The drawing under review shows one solid part. Ordinate dimensions are in mm from its lowest x, y, z. Coordinates: 2 decimals unless noted, no trailing zeros. Order: outer loops, then holes, each group sorted by start corner. A loop starts at its lowest first (then second) coordinate and runs counter-clockwise, first axis right, second up. Notation, with made-up numbers: (4, 69) -> (27, 69) arc R28 cw to (27, 97) -> close; hole circle Ø8 at (-30.5, -22). An arc over 180 degrees is marked (long way). Use a Markdown table: item, result. Add a question column.
Q1. Wall thickness on probe 1 along X at (y, z) = (35.5, 3.75); probe 2 along Y at (x, z) = (56.5, 2.95); probe 3 along Y at (x, z) = (46, 3.3): over which ranges is each line inside the solid? List them lowest first.
Q2. Insertion check: pin 1 (2.5 mm diameter, centred on x = 57, z = 2, fed in from +Y); pin 2 (1 mm diameter, centred on x = 13, z = 3, fed in from +Y); pin 3 (5 mm diameter, centred on x = 29, y = 99, fed in from -Z). Each pin has a flat end and moves straight along its axis. Give the tip position at first contact, or say it passes through.
Q3. Add section A-A (z = 1.45). State the section outline as (x, y) points.
Q4. Add section C-C (x = 35.5). State the section outline as (y, z) points, then the cut area to 3 significant figures.
Q5. Add section B-B (y = 143). State the section outline as (x, z) points, then the cut area to 3 significant figures.
Q6. Add section D-D (x = 45). State the section outline as (y, z) points.
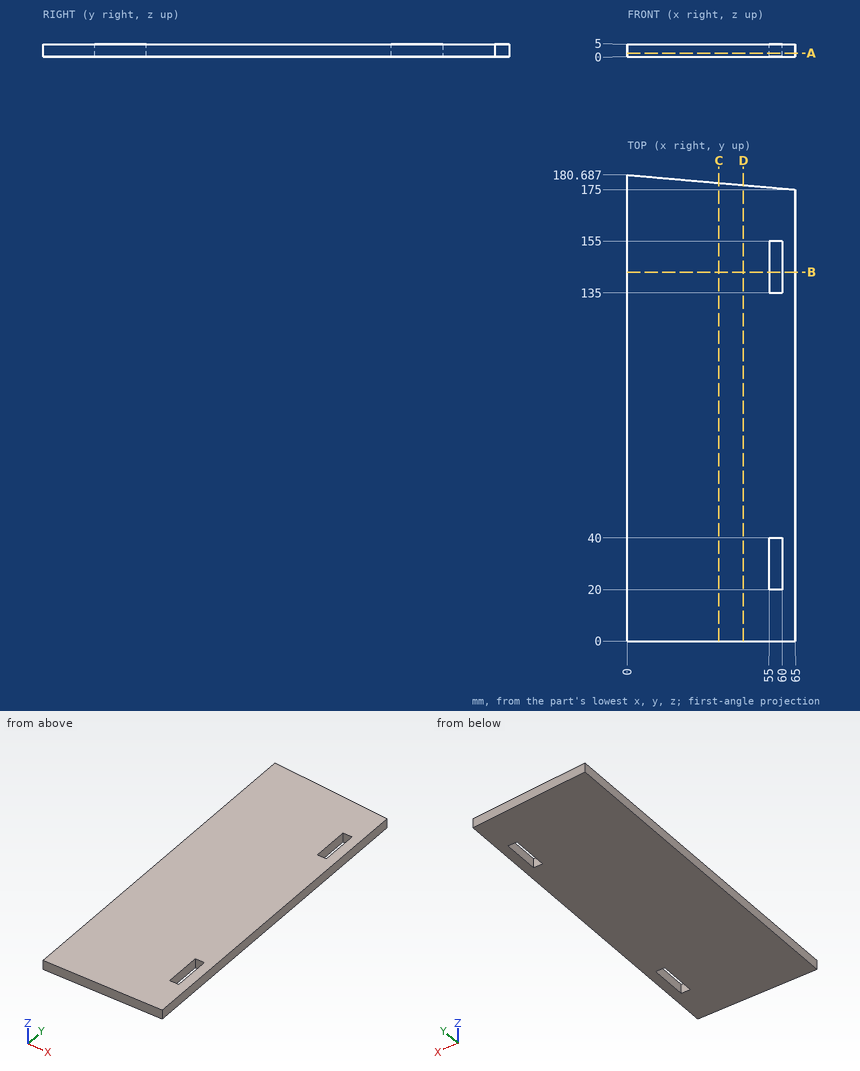
Established:
| question | item | result |
|---|---|---|
| 1 | probe 1 | 0 to 55, 60 to 65 |
| 1 | probe 2 | 0 to 20, 40 to 135, 155 to 175.74 |
| 1 | probe 3 | 0 to 176.66 |
| 2 | pin 1 | y = 175.81 |
| 2 | pin 2 | y = 179.59 |
| 2 | pin 3 | z = 0 |
| 3 | outline | (0, 0) -> (65, 0) -> (65, 175) -> (0, 180.69) -> close; hole (55, 20) -> (60, 20) -> (60, 40) -> (55, 40) -> close; hole (55, 135) -> (60, 135) -> (60, 155) -> (55, 155) -> close |
| 4 | outline | (0, 0) -> (177.58, 0) -> (177.58, 5) -> (0, 5) -> close |
| 4 | area | 888 mm^2 |
| 5 | outline | (0, 0) -> (55, 0) -> (55, 5) -> (0, 5) -> close; (60, 0) -> (65, 0) -> (65, 5) -> (60, 5) -> close |
| 5 | area | 300 mm^2 |
| 6 | outline | (0, 0) -> (176.75, 0) -> (176.75, 5) -> (0, 5) -> close |
